CAD build for the part. Positions are in the model's coordinates, mm. A direction names the side the tool comes from. Give positions to 0.01 mm unless a question says otherwise; leave off trailing zeros. Loops run counter-clockwise (first coordinate to the right, second up) from the corner with the lowest first, then second, coordinate; pieces in that order, holes last.
```python
from build123d import *

# Parameters (mm, degrees)
SKETCH1_W           = 42.3
SKETCH1_H           = 42.3
SKETCH1_R           = 1.5
BOSS_EXTRUDE1_DEPTH = 48
SKETCH2_R           = 4
BOSS_EXTRUDE2_DEPTH = 200


with BuildPart() as part:
    # Sketch1 → Boss-Extrude1 (new body)
    with BuildSketch(Plane.XY):
        Rectangle(SKETCH1_W, SKETCH1_H)
        with Locations((15.5, 15.5)):
            Circle(SKETCH1_R, mode=Mode.SUBTRACT)
        with Locations((-15.5, 15.5)):
            Circle(SKETCH1_R, mode=Mode.SUBTRACT)
        with Locations((-15.5, -15.5)):
            Circle(SKETCH1_R, mode=Mode.SUBTRACT)
        with Locations((15.5, -15.5)):
            Circle(SKETCH1_R, mode=Mode.SUBTRACT)
    extrude(amount=BOSS_EXTRUDE1_DEPTH)

    # Sketch2 → Boss-Extrude2 (add)
    with BuildSketch(Plane.XY.offset(48)):
        with Locations(Location((0, 0, 0), (0, 0, 180))):
            Circle(SKETCH2_R)
    extrude(amount=BOSS_EXTRUDE2_DEPTH)


solid = part.part
```
1. Tool access for faces 1 (the face through (0, 21.15, 24)), 2 (the face through (0.867, 3.905, 146.6)): list every direction of +Z, -Z, +X, -X, +Y, -Y with a clear straight run to the whole face (end or side of a thin tool).
Responses:
face 1: +Z, -Z, +X, -X, +Y
face 2: +Z
2. Probe line 1 along X through (y, z) = (15, 19.5); line 2 along Y through (x, z) = (15.5, 11); line 3 along Z through (x, y) = (-8.5, 19). List the from-to ranges inside material, lowest first.
Responses:
line 1: x = -21.15 to -16.91, -14.09 to 14.09, 16.91 to 21.15
line 2: y = -21.15 to -17, -14 to 14, 17 to 21.15
line 3: z = 0 to 48
3. Saw through at B-B, the plane y = 0. List the corners of the cut face in (x, z), and give its area (3 significant figures).
Responses:
outline: (-21.15, 0) - (21.15, 0) - (21.15, 48) - (4, 48) - (4, 248) - (-4, 248) - (-4, 48) - (-21.15, 48) - close
area: 3,630 mm2
4. Saw through at A-A, the plane z = 25. List the corners of the cut face in (x, y).
Responses:
outline: (-21.15, -21.15) - (21.15, -21.15) - (21.15, 21.15) - (-21.15, 21.15) - close; hole circle Ø3 at (-15.5, -15.5); hole circle Ø3 at (-15.5, 15.5); hole circle Ø3 at (15.5, -15.5); hole circle Ø3 at (15.5, 15.5)
5. Drop flat-ended pins along their axis: pin 1 (6 mm diameter, centred on x = 0.5, z = 77.5, fed in from +Y); pin 2 (4 mm diameter, centred on x = -3, z = 142.5, fed in from -Y); pin 3 (3.5 mm diameter, centred on x = 15.5, y = 15.5, fed in from +Z). Give the stop position or say it passes through.
Responses:
pin 1: stops at y = 4
pin 2: stops at y = -3.87
pin 3: stops at z = 48
6. Saw through at D-D, the plane z = 161. List the corners of the cut face in (x, y).
Responses:
outline: circle Ø8 at (0, 0)
